Check sheet for the modelled part. Datum: model origin and axes. Units: mm. A direction names the side the tool comes from. Round coordinates to 2 decimals unless told otherwise and drop trailing zeros. Write each loop counter-clockwise with the first axis right and the second up, starting at its lowest first coordinate (ties: lowest second). Pieces come first, ordered by that corner, then holes. Notation, with made-up numbers: (46, 30) -> (69, 30) arc R17 cw to (69, 49) -> close; hole circle Ø9 at (-12, 7). An arc over 180 degrees is marked (long way). Use one line per item in the form item = value. Start each with the question number.
Autodesk Inventor part; units mm, degrees
ref_plane "YZ Plane" through (0, 0, 0) normal (1, 0, 0) x (0, 1, 0)
ref_plane "XZ Plane" through (0, 0, 0) normal (0, 1, 0) x (-1, 0, 0)
ref_plane "XY Plane" through (0, 0, 0) normal (0, 0, 1) x (1, 0, 0)
sketch "Sketch1" plane through (0, 0, 0) normal (0, 1, 0) x (-1, 0, 0)
  line L0 (-20, 55.5) -> (20, 55.5)
  line L1 (20, 55.5) -> (20, -55.5)
  line L2 (20, -55.5) -> (-20, -55.5)
  line L3 (-20, -55.5) -> (-20, 55.5)
  line L4 (0, 55.5) -> (0, -55.5) construction
  line L5 (20, 0) -> (-20, 0) construction
  circle A0 centre (9, -44.5) radius 1.8
  circle A1 centre (9, 44.5) radius 1.8
  circle A2 centre (-9, -44.5) radius 1.8
  circle A3 centre (-9, 44.5) radius 1.8
  circle A4 centre (0, 0) radius 2.75
  line L6 (155.5, -20) -> (20, -20)
  line L7 (20, -20) -> (20, 20)
  line L8 (20, 20) -> (155.5, 20)
  line L9 (155.5, 20) -> (155.5, -20)
  point P0 (145, 0)
  point P1 (145, -20)
  dimension "d0" = 40
  dimension "d1" = 111
  dimension "d2" = 3.6
  dimension "d3" = 5.5
  dimension "d4" = 40
extrude "Extrusion1" add sketch "Sketch1" along normal blind 10
sketch "Sketch2" plane through (0, 10, 0) normal (0, 1, 0) x (1, 0, 0)
  circle A0 centre (-9, 44.5) radius 1.8
  circle A1 centre (-9, 44.5) radius 3.25
  circle A2 centre (9, 44.5) radius 1.8
  circle A3 centre (9, 44.5) radius 3.25
  circle A4 centre (9, -44.5) radius 1.8
  circle A5 centre (9, -44.5) radius 3.25
  circle A6 centre (-9, -44.5) radius 1.8
  circle A7 centre (-9, -44.5) radius 3.25
  point P0 (0, 0)
  dimension "d7" = 6.5
  dimension "d8" = 6.5
  dimension "d9" = 6.5
  dimension "d10" = 6.5
extrude "Extrusion2" cut sketch "Sketch2" against normal blind 4
fillet "Fillet1" radius 1 4 edges at (-12.25, 10, 44.5) (5.75, 10, 44.5) (5.75, 10, -44.5) (-12.25, 10, -44.5)
fillet "Fillet2" radius 20 2 edges at (-20, 5, 20) (-20, 5, -20)
sketch "Sketch3" plane through (-155.5, 0, 20) normal (0, 0, 1) x (1, 0, 0)
  line L0 (0, 0) -> (0, 10)
  line L1 (0, 10) -> (-25, 10)
  line L2 (-25, 10) -> (-25, 5)
  line L3 (-25, 5) -> (0, 5)
  line L4 (0, 5) -> (0, 10)
  line L5 (0, 5) -> (15, 5)
  line L6 (15, 5) -> (15, 0)
  line L7 (15, 0) -> (0, 0)
  line L8 (0, 0) -> (0, 5)
  point P0 (155.5, 0)
  dimension "d15" = 25
  dimension "d16" = 5
  dimension "d17" = 15
  dimension "d18" = 5
extrude "Extrusion3" add sketch "Sketch3" against normal blind 40 contours L3 L2 L1 L0
extrude "Extrusion4" cut sketch "Sketch3" against normal blind 40 contours L0 L5 L6 L7
sketch "Sketch4" plane through (0, 10, 0) normal (0, 1, 0) x (1, 0, 0)
  circle A0 centre (0, 0) radius 2.75 construction
  circle A1 centre (-9, 44.5) radius 1.8 construction
  circle A2 centre (9, 44.5) radius 1.8 construction
  line L0 (-9, 44.5) -> (9, 44.5) construction
  line L1 (0, 29.5) -> (0, 15) construction
  line L2 (-5, 29.5) -> (-5, 15)
  line L3 (5, 15) -> (5, 29.5)
  arc A3 (5, 29.5) -> (-5, 29.5) centre (0, 29.5) ccw
  arc A4 (-5, 15) -> (5, 15) centre (0, 15) ccw
  line L4 (-7.5, 0) -> (7.5, 0) construction
  line L5 (-5, -29.5) -> (-5, -15)
  line L6 (5, -15) -> (5, -29.5)
  arc A5 (-5, -29.5) -> (5, -29.5) centre (0, -29.5) ccw
  arc A6 (5, -15) -> (-5, -15) centre (0, -15) ccw
  line L7 (-160.5, 0) -> (0, 0) construction
  line L8 (-40, 20) -> (-140.5, 20) construction
  line L9 (-140.5, -20) -> (-140.5, 20) construction
  line L10 (-140.5, 20) -> (-140.5, -20) construction
  point P0 (0, 22.25)
  point P1 (-95.25, 0)
  point P2 (-65.25, 0)
  point P3 (-15, 0)
  point P4 (-125.5, 0)
  dimension "d33" = 10
  dimension "d34" = 15
extrude "Extrusion5" cut sketch "Sketch4" against normal blind 10
sketch "Sketch5" plane through (-40, 0, 20) normal (0, 0, 1) x (1, 0, 0)
  line L0 (0, 10) -> (-140.5, 10)
  line L1 (-140.5, 10) -> (-155.5, 10)
  line L2 (-155.5, 10) -> (-155.5, 5)
  line L3 (-155.5, 5) -> (-140.5, 5)
  line L4 (-140.5, 5) -> (-140.5, 10)
  line L5 (-100.5, 0) -> (-100.5, 5)
  line L6 (-100.5, 5) -> (-115.5, 5)
  line L7 (-115.5, 5) -> (-115.5, 0)
  line L8 (-115.5, 0) -> (-100.5, 0)
  line L9 (-100.5, 0) -> (-100.5, 5)
  point P0 (40, 0)
  dimension "d49" = 15
  dimension "d53" = 15
  dimension "d54" = 5
extrude "Extrusion6" add sketch "Sketch5" against normal blind 40
sketch "Sketch6" plane through (0, 10, 0) normal (0, 1, 0) x (1, 0, 0)
  circle A0 centre (-175.5, 0) radius 2.75
  line L0 (-175.5, 0) -> (0, 0) construction
  circle A1 centre (-87.75, 0) radius 2.75
  line L1 (-155.5, -20) -> (-155.5, 20) construction
  line L2 (-155.5, -20) -> (-155.5, 20) construction
  line L3 (-140.5, 0) -> (-102.75, 0) construction
  line L4 (-140.5, -5) -> (-102.75, -5)
  line L5 (-102.75, 5) -> (-140.5, 5)
  arc A2 (-140.5, 5) -> (-140.5, -5) centre (-140.5, 0) ccw
  arc A3 (-102.75, -5) -> (-102.75, 5) centre (-102.75, 0) ccw
  line L6 (-72.75, 0) -> (-15, 0) construction
  line L7 (-72.75, -5) -> (-15, -5)
  line L8 (-15, 5) -> (-72.75, 5)
  arc A4 (-72.75, 5) -> (-72.75, -5) centre (-72.75, 0) ccw
  arc A5 (-15, -5) -> (-15, 5) centre (-15, 0) ccw
  point P0 (-155.5, 0)
  point P1 (-121.625, 0)
  point P2 (-43.875, 0)
  dimension "d55" = 5.5
  dimension "d58" = 87.75
  dimension "d63" = 10
  dimension "d64" = 10
extrude "Extrusion7" cut sketch "Sketch6" against normal through all
sketch "Sketch8" plane through (0, 10, 0) normal (0, 1, 0) x (1, 0, 0)
  circle A0 centre (-87.75, 0) radius 2.75
  line L0 (-87.75, -20) -> (-87.75, 20) construction
  line L1 (-40, 20) -> (-155.5, 20)
  line L2 (-107.75, 20) -> (-67.75, 20) construction
  line L3 (-107.75, -20) -> (-67.75, -20) construction
  line L4 (-155.5, -20) -> (-40, -20) construction
  line L5 (-107.75, 20) -> (-67.75, 20)
  line L6 (-67.75, 20) -> (-67.75, 65.5)
  line L7 (-67.75, 65.5) -> (-107.75, 65.5)
  line L8 (-107.75, 65.5) -> (-107.75, 20)
  line L9 (-107.75, -20) -> (-67.75, -20)
  line L10 (-67.75, -20) -> (-67.75, -65.5)
  line L11 (-67.75, -65.5) -> (-107.75, -65.5)
  line L12 (-107.75, -65.5) -> (-107.75, -20)
  point P0 (0, 0)
  dimension "d67" = 40
  dimension "d68" = 40
  dimension "d69" = 45.5
  dimension "d70" = 45.5
extrude "Extrusion8" add sketch "Sketch8" against normal blind 10 contours L1 L8 L7 L6 | L9 L10 L11 L12
sketch "Sketch9" plane through (0, 10, 0) normal (0, 1, 0) x (1, 0, 0)
  circle A0 centre (-87.75, 0) radius 2.75 construction
  line L0 (20, 0) -> (-195.5, 0) construction
  line L1 (-195.5, -20) -> (-195.5, 20) construction
  line L2 (-87.75, -65.5) -> (-87.75, 65.5) construction
  line L3 (-107.75, 65.5) -> (-67.75, 65.5) construction
  circle A1 centre (-87.75, -45.5) radius 2.75
  circle A2 centre (-87.75, 45.5) radius 2.75
  line L4 (-87.75, -30.5) -> (-87.75, -15) construction
  line L5 (-82.75, -30.5) -> (-82.75, -15)
  line L6 (-92.75, -15) -> (-92.75, -30.5)
  arc A3 (-92.75, -30.5) -> (-82.75, -30.5) centre (-87.75, -30.5) ccw
  arc A4 (-82.75, -15) -> (-92.75, -15) centre (-87.75, -15) ccw
  line L7 (-87.75, 15) -> (-87.75, 30.5) construction
  line L8 (-82.75, 15) -> (-82.75, 30.5)
  line L9 (-92.75, 30.5) -> (-92.75, 15)
  arc A5 (-92.75, 15) -> (-82.75, 15) centre (-87.75, 15) ccw
  arc A6 (-82.75, 30.5) -> (-92.75, 30.5) centre (-87.75, 30.5) ccw
  point P0 (0, 0)
  point P1 (-87.75, -22.75)
  point P2 (-87.75, 22.75)
  dimension "d74" = 5.5
  dimension "d75" = 10
  dimension "d76" = 10
extrude "Extrusion9" cut sketch "Sketch9" against normal blind 10
fillet "Fillet4" radius 20 4 edges at (-67.75, 5, 20) (-67.75, 5, -20) (-107.75, 5, -20) (-107.75, 5, 20)
fillet "Fillet5" radius 10 4 edges at (-67.75, 5, 65.5) (-107.75, 5, 65.5) (-107.75, 5, -65.5) (-67.75, 5, -65.5)
sketch "Sketch11" plane through (-195.5, 5, 20) normal (0, -1, 0) x (1, 0, 0)
  line L0 (67.75, 0) -> (0, 0)
  line L1 (40, 0) -> (40, -40)
  line L2 (0, 0) -> (40, 0)
  line L3 (40, 0) -> (40, -40)
  line L4 (40, -40) -> (0, -40)
  line L5 (0, -40) -> (0, 0)
  line L6 (0, 0) -> (40, 0)
  line L7 (40, 0) -> (40, -0.15)
  line L8 (40, -0.15) -> (0, -0.15)
  line L9 (0, -0.15) -> (0, 0)
  line L10 (0, -40) -> (40, -40)
  line L11 (40, -40) -> (40, -39.85)
  line L12 (40, -39.85) -> (0, -39.85)
  line L13 (0, -39.85) -> (0, -40)
  point P0 (195.5, -20)
  point P1 (0, -0.15)
  point P2 (40, -0.15)
  dimension "d81" = 40
  dimension "d82" = 0.15
  dimension "d83" = 40
  dimension "d84" = 0.15
extrude "Extrusion10" cut sketch "Sketch11" against normal through all contours L1 L8 L5 L0 | L1 L4 L5 L12
properties part number "Chassis Front Spine"
1. Sectioned sample at B-B (x = -87.75). Enter the section's corners in (y, z), and give its area (3 significant figures).
2. Sectioned sample at C-C (y = 2). Give the number of separate pieces and of enclosed holes in the cut face, and give its area (3 significant figures).
3. Scan lines: probe 1 along Z at (x, y) = (9, 7.1); probe 2 along Z at (x, y) = (-9, 3.15); probe 3 along X at (y, z) = (6.25, 45.5). Record each from-to range of solid material in increasing order.
4. Depth check by flat-ended pin: pin 1 (2 mm diameter, centred on x = 8.5, z = 44.5, fed in from +Y); pin 2 (5 mm diameter, centred on x = -10, z = 44.5, fed in from +Y); pin 3 (1 mm diameter, centred on x = -141, y = 4, fed in from -Z); pin 4 (3 mm diameter, centred on y = 3.5, z = -48.5, fed in from -X). Enter the tip coordinate at first touch or a pass-through.
5. Mould release check, pull along Z, two halves, no side actions. Record for faces 5 (the face through (-107.75, 5, -48)), 6 (the face through (-175, 7, -19.85)), 7 (the face through (10.4, 6, 45.9)): +Z half, -Z half, draft (parallel to the pull), parting line (faces both ways), or undercut.
6. Tool access check on faces 1 (the face through (-5, 5, -22)), 2 (the face through (10.4, 6, -43.1)), 3 (the face through (-44, 5, 20)), 4 (the face through (-26.014, 5.07, -25.703)). Record the directions out of +Z, -Z, +X, -X, +Y, -Y that give a thin tool (end or side, any length) a straight path to the whole face; none if there is none.
7. Sectioned sample at A-A (x = 0). Enter the section's corners in (y, z).
Returned:
q1.outline = (0, -65.5) -> (10, -65.5) -> (10, -48.25) -> (0, -48.25) -> close; (0, -42.75) -> (10, -42.75) -> (10, -35.5) -> (0, -35.5) -> close; (0, -10) -> (10, -10) -> (10, -2.75) -> (0, -2.75) -> close; (0, 2.75) -> (10, 2.75) -> (10, 10) -> (0, 10) -> close; (0, 35.5) -> (10, 35.5) -> (10, 42.75) -> (0, 42.75) -> close; (0, 48.25) -> (10, 48.25) -> (10, 65.5) -> (0, 65.5) -> close
q1.area = 635 mm^2
q2.separate_pieces = 1
q2.enclosed_holes = 14
q2.area = 11,800 mm^2
q3.probe_1 = -55.5 to -47.75, -41.25 to 41.25, 47.75 to 55.5
q3.probe_2 = -55.5 to -46.3, -42.7 to 42.7, 46.3 to 55.5
q3.probe_3 = -107.75 to -90.5, -85 to -67.75, -20 to -12.09, -5.91 to 5.91, 12.09 to 20
q4.pin_1 = through
q4.pin_2 = 9.66
q4.pin_3 = -20
q4.pin_4 = -107.75
q5.face_5 = draft
q5.face_6 = -Z half
q5.face_7 = undercut
q6.face_1 = +Y, -Y
q6.face_2 = +Y
q6.face_3 = +Z, +Y, -Y
q6.face_4 = -Z, +Y, -Y
q7.outline = (0, -55.5) -> (10, -55.5) -> (10, -34.5) -> (0, -34.5) -> close; (0, -10) -> (10, -10) -> (10, -2.75) -> (0, -2.75) -> close; (0, 2.75) -> (10, 2.75) -> (10, 10) -> (0, 10) -> close; (0, 34.5) -> (10, 34.5) -> (10, 55.5) -> (0, 55.5) -> close
